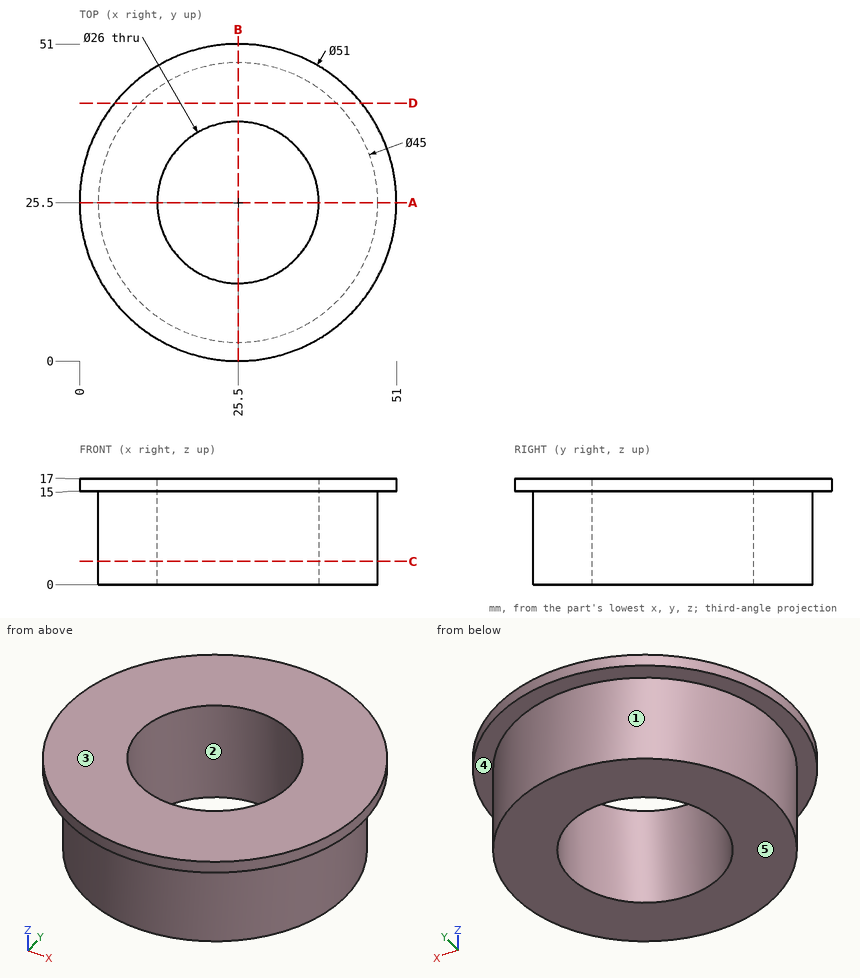
Design review of the part shown in the three views and the two pictorial views. Dimensions are in mm from the part's minimum x, y and z. A direction names the side the tool comes from. Coordinates: 2 decimals unless noted, no trailing zeros. Order: outer loops, then holes, each group sorted by start corner. A loop starts at its lowest first (then second) coordinate and runs counter-clockwise, first axis right, second up.
Item 1: Take a section at C-C, the plane z = 3.75. Write out the cut boundary in (x, y).
Item 2: The part is to be moulded in two halves that separate along X. For the marked faces 1, 2 and 3, say which applies: pulls with the +X half, pulls with the -X half, needs draft (parallel to the pull), parting line crosses it, or undercut.
Item 3: For the marked faces 4 and 5, list the 3-axis set-ups (+Z, -Z, +X, -X, +Y, -Y) from which the entire face can be reached by the end or side of a thin tool; tool diameter is ignored.
Item 4: Take a section at D-D, the plane y = 41.5. Write out the cut boundary in (x, z).
Item 5: Take a section at A-A, the plane y = 25.5. Write out the cut boundary in (x, z), then the cut area to 3 significant figures.
Item 6: For pin 1 Ø8 at (y, z) = (42, 5) entering from -X; pin 2 Ø6 at (x, z) = (46, 11.5) entering from -Y; pin 3 Ø15.5 at (x, y) = (25.5, 25.5) entering from +Z; pin 4 Ø1 at (x, z) = (35, 9) entering from +Y, all flat-tipped, find the tip position at first contact; note any pin that passes through.
Item 7: For line 1 (Y direction, x = 25.5, z = 13.25); line 2 (Y direction, x = 18.5, z = 2.75); line 3 (X direction, y = 26.5, z = 7.75), list the stretches that pass through material, from the lowest coordinate up.
The answers:
1. outline: circle Ø45 at (25.5, 25.5); hole circle Ø26 at (25.5, 25.5)
2. face 1: parting line crosses it
2. face 2: undercut
2. face 3: needs draft
3. face 4: -Z
3. face 5: -Z, +X, -X, +Y, -Y
4. outline: (5.64, 15) - (9.68, 15) - (9.68, 0) - (41.32, 0) - (41.32, 15) - (45.36, 15) - (45.36, 17) - (5.64, 17) - close
5. outline: (0, 15) - (3, 15) - (3, 0) - (12.5, 0) - (12.5, 17) - (0, 17) - close; (38.5, 0) - (48, 0) - (48, 15) - (51, 15) - (51, 17) - (38.5, 17) - close
5. area: 335 mm2
6. pin 1: stops at x = 6.79
6. pin 2: stops at y = 11.36
6. pin 3: passes through
6. pin 4: stops at y = 46.12
7. line 1: y = 3 to 12.5, 38.5 to 48
7. line 2: y = 4.12 to 14.55, 36.45 to 46.88
7. line 3: x = 3.02 to 12.54, 38.46 to 47.98
